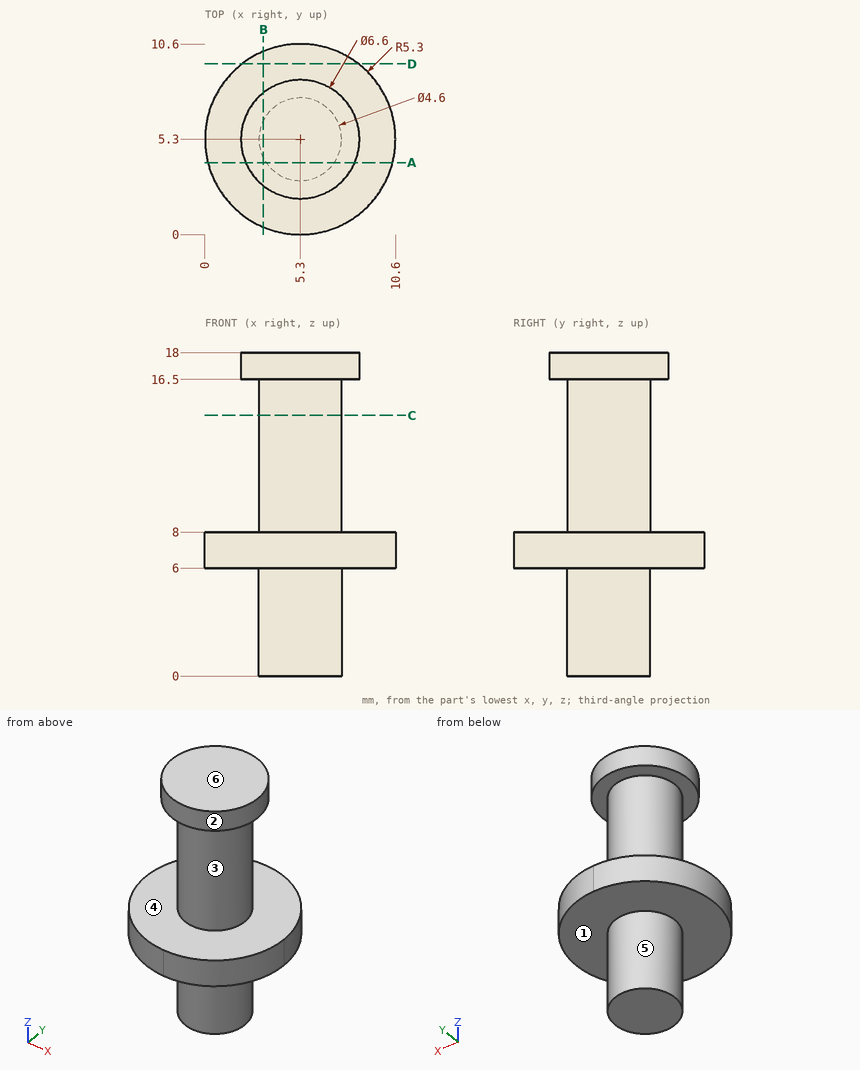
Verification items for this drawing (mm, ordinates from the low corner). A direction names the side the tool comes from. Round coordinates to 2 decimals unless told otherwise and drop trailing zeros. Loops run counter-clockwise (first coordinate to the right, second up) from the corner with the lowest first, then second, coordinate; pieces in that order, holes last. Notation, with made-up numbers: (-1, 82.5) - (46, 82.5) arc R24 ccw to (46, 103.5) - close; hole circle Ø2 at (9.5, 9.25). An arc over 180 degrees is marked (long way). Answer as CSV lines item,"result". Start each with the question number.
Item 1: Release check for a two-part mould opening along Z. For the marked faces 1, 2 and 3 record: +Z half, -Z half, draft (parallel to the pull), parting line (faces both ways), or undercut.
Item 2: Scan lines: line 1 (Z direction, x = 3, y = 7.5); line 2 (Z direction, x = 0.75, y = 7.5); line 3 (Y direction, x = 3.5, z = 10.5). Record each from-to range of solid material in increasing order. Write a range as [from, to].
Item 3: Section check D-D (y = 9.5). Record the boundary of the cut face in (x, z).
Item 4: Section check B-B (x = 3.25). Record the boundary of the cut face in (y, z).
Item 5: Section check A-A (y = 4). Record the boundary of the cut face in (x, z).
Item 6: Depth check by flat-ended pin: P1, Ø1.5, axis at x = 4, z = 3.5, coming from the +Y side; P2, Ø4, axis at x = 9.5, y = 3.5, coming from the -Z side; P3, Ø3, axis at y = 3.5, z = 12.5, coming from the -X side; P4, Ø3, axis at x = 7, y = 3, coming from the -Z side. Enter the tip coordinate at first touch or a pass-through.
Item 7: Section check C-C (z = 14.5). Record the boundary of the cut face in (x, y), and give its area (3 significant figures).
Item 8: Set-up check for the marked faces 4, 5 and 6: record each of +Z, -Z, +X, -X, +Y, -Y from which the full face is reachable in a straight line by a thin tool's end or side.
Report:
1,face 1,"-Z half"
1,face 2,"draft"
1,face 3,"undercut"
2,line 1,"z = [6, 8], [16.5, 18]"
2,line 2,"z = [6, 8]"
2,line 3,"y = [3.87, 6.73]"
3,outline,"(2.07, 6) - (8.53, 6) - (8.53, 8) - (2.07, 8) - close"
4,outline,"(0.41, 6) - (4.26, 6) - (4.26, 0) - (6.34, 0) - (6.34, 6) - (10.19, 6) - (10.19, 8) - (6.34, 8) - (6.34, 16.5) - (7.89, 16.5) - (7.89, 18) - (2.71, 18) - (2.71, 16.5) - (4.26, 16.5) - (4.26, 8) - (0.41, 8) - close"
5,outline,"(0.16, 6) - (3.4, 6) - (3.4, 0) - (7.2, 0) - (7.2, 6) - (10.44, 6) - (10.44, 8) - (7.2, 8) - (7.2, 16.5) - (8.33, 16.5) - (8.33, 18) - (2.27, 18) - (2.27, 16.5) - (3.4, 16.5) - (3.4, 8) - (0.16, 8) - close"
6,P1,"stops at y = 7.53"
6,P2,"stops at z = 6"
6,P3,"stops at x = 3.02"
6,P4,"stops at z = 0"
7,outline,"circle Ø4.6 at (5.3, 5.3)"
7,area,"16.6 mm2"
8,face 4,"none"
8,face 5,"-Z"
8,face 6,"+Z, +X, -X, +Y, -Y"
